Check sheet for the modelled part. Datum: model origin and axes. Units: mm. A direction names the side the tool comes from. Coordinates: 2 decimals unless noted, no trailing zeros. Loops run counter-clockwise (first coordinate to the right, second up) from the corner with the lowest first, then second, coordinate; pieces in that order, holes last. Notation, with made-up numbers: M 78,-18 L 135,-18 A19 ccw 135,19 Z; hole C 24,27.5 d11. An arc over 180 degrees is marked long. Answer in a Markdown table with one row per item. Add a question column.
```python
from build123d import *

# Parameters (mm, degrees)
ESQUISSE1_W       = 5.08
ESQUISSE1_H       = 2.54
EXTRUSION1_DEPTH  = 4
ESQUISSE2_R       = 0.915
EXTRUSION2_DEPTH  = 0.4
ESQUISSE3_R       = 0.535
EXTRUSION3_DEPTH  = 1.565
D_ME1_FACE_RADIUS = 0.535
D_ME1_HEIGHT      = 0.535
D_ME2_FACE_RADIUS = 0.535
D_ME2_HEIGHT      = 0.535
ESQUISSE4_R       = 0.4
EXTRUSION4_DEPTH  = 3


with BuildPart() as part:
    # Esquisse1 → Extrusion1 (new body)
    with BuildSketch(Plane.XY):
        with Locations((2.54, 1.27)):
            Rectangle(ESQUISSE1_W, ESQUISSE1_H)
    extrude(amount=EXTRUSION1_DEPTH)

    # Esquisse2 → Extrusion2 (add)
    with BuildSketch(Plane.XY.offset(4)):
        with Locations(Location((3.81, 1.27, 0), (0, 0, 180))):
            Circle(ESQUISSE2_R)
        with Locations(Location((1.27, 1.27, 0), (0, 0, 180))):
            Circle(ESQUISSE2_R)
    extrude(amount=EXTRUSION2_DEPTH)

    # Esquisse3 → Extrusion3 (add)
    with BuildSketch(Plane(origin=(0, 0, 0), x_dir=(-1, 0, 0), z_dir=(0, 0, -1))):
        with Locations((-3.81, 1.27)):
            Circle(ESQUISSE3_R)
        with Locations((-1.27, 1.27)):
            Circle(ESQUISSE3_R)
    extrude(amount=EXTRUSION3_DEPTH)

    # Dôme1: a dome of height H over a round flat face of radius A is a cap of a sphere of radius (A * A + H * H) / (2 * H)
    d_me1_r = (D_ME1_FACE_RADIUS * D_ME1_FACE_RADIUS + D_ME1_HEIGHT * D_ME1_HEIGHT) / (2 * D_ME1_HEIGHT)
    d_me1_base = Plane((3.81, 1.27, -1.565), z_dir=(0, 0, -1))
    with Locations(d_me1_base.offset(D_ME1_HEIGHT - d_me1_r)):
        d_me1_ball = Sphere(d_me1_r, mode=Mode.PRIVATE)
    add(split(d_me1_ball, bisect_by=d_me1_base, keep=Keep.TOP, mode=Mode.PRIVATE))

    # Dôme2: a dome of height H over a round flat face of radius A is a cap of a sphere of radius (A * A + H * H) / (2 * H)
    d_me2_r = (D_ME2_FACE_RADIUS * D_ME2_FACE_RADIUS + D_ME2_HEIGHT * D_ME2_HEIGHT) / (2 * D_ME2_HEIGHT)
    d_me2_base = Plane((1.27, 1.27, -1.565), z_dir=(0, 0, -1))
    with Locations(d_me2_base.offset(D_ME2_HEIGHT - d_me2_r)):
        d_me2_ball = Sphere(d_me2_r, mode=Mode.PRIVATE)
    add(split(d_me2_ball, bisect_by=d_me2_base, keep=Keep.TOP, mode=Mode.PRIVATE))

    # Esquisse4 → Extrusion4 (add)
    with BuildSketch(Plane.XY.offset(4.4)):
        with Locations((3.81, 1.27)):
            Circle(ESQUISSE4_R)
        with Locations((1.27, 1.27)):
            Circle(ESQUISSE4_R)
    extrude(amount=EXTRUSION4_DEPTH)


solid = part.part
```
Q1. Access from +Z, -Z, +X, -X, +Y, -Y to the whole of each face (thin tool, end or side, straight path). Record for faces 4 (the face through (3, 2.54, 2)), 5 (the face through (3.316, 1.065, -0.772)), 6 (the face through (3.388, 2.082, 4.197)).
Q2. Cross-section at D-D (z = -1). Record the cut outline in (x, y) (3 decimals), plus the area to 3 significant figures.
Q3. Mould release check, pull along X, two halves, no side actions. Record for faces 1 (the face through (3, 1, 0)), 2 (the face through (3, 0, 2)), 3 (the face through (0, 1, 2)): released by +X, released by -X, zero draft, split by the parting line, or undercut.
Q4. Cross-section at B-B (x = 3.81). Record the cut outline in (y, z) (3 decimals).
Q5. Cross-section at C-C (z = 4.5). Record the cut outline in (x, y), plus the area to 3 significant figures.
Q6. Go/stop test with flat-tipped pins: pin 1 (0.8 mm diameter, centred on x = 3, y = 1.5, fed in from +Z); pin 2 (1.3 mm diameter, centred on x = 2, y = 1, fed in from -Z). Record where each tip stops, or that it passes through.
Q7. Cross-section at A-A (y = 1.27). Record the cut outline in (x, z) (3 decimals), plus the area to 3 significant figures.
Q8. Thickness scan on L1, parallel to Z at x = 0.5, y = 2.1; L2, parallel to X at y = 0.9, z = -0.5; L3, parallel to Z at x = 3.5, y = 1.95. Record the ranges inside material, lowest first.
Answer key:
| question | item | result |
|---|---|---|
| 1 | face 4 | +Z, -Z, +X, -X, +Y |
| 1 | face 5 | -Z |
| 1 | face 6 | +Z |
| 2 | outline | C 1.27,1.27 d1.07; C 3.81,1.27 d1.07 |
| 2 | area | 1.80 mm^2 |
| 3 | face 1 | undercut |
| 3 | face 2 | zero draft |
| 3 | face 3 | released by -X |
| 4 | outline | M 0,0 L 0.735,0 L 0.735,-1.565 A0.535 ccw 1.805,-1.565 L 1.805,0 L 2.54,0 L 2.54,4 L 2.185,4 L 2.185,4.4 L 1.67,4.4 L 1.67,7.4 L 0.87,7.4 L 0.87,4.4 L 0.355,4.4 L 0.355,4 L 0,4 Z |
| 5 | outline | C 1.27,1.27 d0.8; C 3.81,1.27 d0.8 |
| 5 | area | 1.01 mm^2 |
| 6 | pin 1 | z = 4.4 |
| 6 | pin 2 | z = -2.08 |
| 7 | outline | M 0,0 L 0.735,0 L 0.735,-1.565 A0.535 ccw 1.805,-1.565 L 1.805,0 L 3.275,0 L 3.275,-1.565 A0.535 ccw 4.345,-1.565 L 4.345,0 L 5.08,0 L 5.08,4 L 4.725,4 L 4.725,4.4 L 4.21,4.4 L 4.21,7.4 L 3.41,7.4 L 3.41,4.4 L 2.895,4.4 L 2.895,4 L 2.185,4 L 2.185,4.4 L 1.67,4.4 L 1.67,7.4 L 0.87,7.4 L 0.87,4.4 L 0.355,4.4 L 0.355,4 L 0,4 Z |
| 7 | area | 30.8 mm^2 |
| 8 | L1 | 0 to 4 |
| 8 | L2 | 0.88 to 1.66, 3.42 to 4.2 |
| 8 | L3 | 0 to 4.4 |
